```python
from build123d import *

# Parameters (mm, degrees)
F0_R     = 3
F0_R_2   = 7.5
F1_DEPTH = 25
F3_ANGLE = 20


with BuildPart() as f1:
    # F0 (on Top) → F1 (new body)
    with BuildSketch(Plane.XY):
        with BuildLine():
            Line((3, 24.819347), (2, 29.933259))
            Line((2, 29.933259), (-2, 29.933259))
            Line((-2, 29.933259), (-3, 24.819347))
            ThreePointArc((-3, 24.819347), (-4.877258, 24.519632), (-6.726314, 24.078137))
            Line((-6.726314, 24.078137), (-9.607203, 28.420092))
            Line((-9.607203, 28.420092), (-13.302721, 26.889359))
            Line((-13.302721, 26.889359), (-12.269592, 21.782037))
            ThreePointArc((-12.269592, 21.782037), (-13.889256, 20.78674), (-15.428608, 19.671249))
            Line((-15.428608, 19.671249), (-19.751797, 22.580224))
            Line((-19.751797, 22.580224), (-22.580224, 19.751797))
            Line((-22.580224, 19.751797), (-19.671249, 15.428609))
            ThreePointArc((-19.671249, 15.428609), (-20.78674, 13.889256), (-21.782037, 12.269592))
            Line((-21.782037, 12.269592), (-26.889359, 13.302722))
            Line((-26.889359, 13.302722), (-28.420092, 9.607203))
            Line((-28.420092, 9.607203), (-24.078137, 6.726315))
            ThreePointArc((-24.078137, 6.726315), (-24.519632, 4.877258), (-24.819347, 3))
            Line((-24.819347, 3), (-29.933259, 2))
            Line((-29.933259, 2), (-29.933259, -2))
            Line((-29.933259, -2), (-24.819347, -3))
            ThreePointArc((-24.819347, -3), (-24.519632, -4.877258), (-24.078137, -6.726314))
            Line((-24.078137, -6.726314), (-28.420092, -9.607203))
            Line((-28.420092, -9.607203), (-26.889359, -13.302721))
            Line((-26.889359, -13.302721), (-21.782037, -12.269592))
            ThreePointArc((-21.782037, -12.269592), (-20.78674, -13.889256), (-19.671249, -15.428608))
            Line((-19.671249, -15.428608), (-22.580224, -19.751797))
            Line((-22.580224, -19.751797), (-19.751797, -22.580224))
            Line((-19.751797, -22.580224), (-15.428608, -19.671249))
            ThreePointArc((-15.428608, -19.671249), (-13.889256, -20.78674), (-12.269592, -21.782037))
            Line((-12.269592, -21.782037), (-13.302721, -26.889359))
            Line((-13.302721, -26.889359), (-9.607203, -28.420092))
            Line((-9.607203, -28.420092), (-6.726314, -24.078137))
            ThreePointArc((-6.726314, -24.078137), (-4.877258, -24.519632), (-3, -24.819347))
            Line((-3, -24.819347), (-2, -29.933259))
            Line((-2, -29.933259), (2, -29.933259))
            Line((2, -29.933259), (3, -24.819347))
            ThreePointArc((3, -24.819347), (4.877258, -24.519632), (6.726314, -24.078137))
            Line((6.726314, -24.078137), (9.607203, -28.420092))
            Line((9.607203, -28.420092), (13.302721, -26.889359))
            Line((13.302721, -26.889359), (12.269592, -21.782037))
            ThreePointArc((12.269592, -21.782037), (13.889256, -20.78674), (15.428608, -19.671249))
            Line((15.428608, -19.671249), (19.751797, -22.580224))
            Line((19.751797, -22.580224), (22.580224, -19.751797))
            Line((22.580224, -19.751797), (19.671249, -15.428608))
            ThreePointArc((19.671249, -15.428608), (20.78674, -13.889256), (21.782037, -12.269592))
            Line((21.782037, -12.269592), (26.889359, -13.302721))
            Line((26.889359, -13.302721), (28.420092, -9.607203))
            Line((28.420092, -9.607203), (24.078137, -6.726314))
            ThreePointArc((24.078137, -6.726314), (24.519632, -4.877258), (24.819347, -3))
            Line((24.819347, -3), (29.933259, -2))
            Line((29.933259, -2), (29.933259, 2))
            Line((29.933259, 2), (24.819347, 3))
            ThreePointArc((24.819347, 3), (24.519632, 4.877258), (24.078137, 6.726314))
            Line((24.078137, 6.726314), (28.420092, 9.607203))
            Line((28.420092, 9.607203), (26.889359, 13.302721))
            Line((26.889359, 13.302721), (21.782037, 12.269592))
            ThreePointArc((21.782037, 12.269592), (20.78674, 13.889256), (19.671249, 15.428608))
            Line((19.671249, 15.428608), (22.580224, 19.751797))
            Line((22.580224, 19.751797), (19.751797, 22.580224))
            Line((19.751797, 22.580224), (15.428608, 19.671249))
            ThreePointArc((15.428608, 19.671249), (13.889256, 20.78674), (12.269592, 21.782037))
            Line((12.269592, 21.782037), (13.302721, 26.889359))
            Line((13.302721, 26.889359), (9.607203, 28.420092))
            Line((9.607203, 28.420092), (6.726314, 24.078137))
            ThreePointArc((6.726314, 24.078137), (4.877258, 24.519632), (3, 24.819347))
        make_face()
        with Locations((5.212864, -15)):
            Circle(F0_R, mode=Mode.SUBTRACT)
        Circle(F0_R_2, mode=Mode.SUBTRACT)
        with Locations((0, 15)):
            Circle(F0_R, mode=Mode.SUBTRACT)
    extrude(amount=F1_DEPTH)


with BuildPart() as f1_1:
    # F3: moved
    add(f1.part.rotate(Axis((0.748886, 0, 25), (1, 0, 0)), F3_ANGLE))


solid = f1_1.part
```
Model file for the job. Use its own axes, mm. A direction names the side the tool comes from. Give positions to 0.01 mm unless a question says otherwise; leave off trailing zeros. Loops run counter-clockwise (first coordinate to the right, second up) from the corner with the lowest first, then second, coordinate; pieces in that order, holes last. Notation, with made-up numbers: M 89.5,28.5 L 138.5,28.5 A25 ccw 138.5,56.5 Z; hole C 86,67.25 d9. An arc over 180 degrees is marked long. Use one line per item in the form item = value.
Item 1: Slice it at A-A on x = 10.5. List the corners of the cut face in (y, z).
Filled in:
outline = M -26.36,15.41 L -17.81,-8.09 L 34.91,11.1 L 26.36,34.59 Z
Item 2: Which spindle directions (+Z, -Z, +X, -X, +Y, -Y) get a long thin tool onto all of the face, cutting with end or side? Do faces 4 (the flat face through (26.22, 11.99, 15.88)), 5 (the cylindrical face through (-4.85, 27.38, 21.48)), 6 (the flat face through (-27.34, 6.69, 13.95)). Say none if no direction does.
Filled in:
face_4 = +X
face_5 = +Z, +Y
face_6 = -X
Item 3: Two-plate mould, pull along X, no slides. Class faces 1 (the flat face through (-27.644, 15.124, 17.016)), 2 (the flat face through (29.933, 4, 13)), 3 (the flat face through (8.147, -20.302, 4.122)): released by +X, released by -X, zero draft, split by the parting line, or undercut.
Filled in:
face_1 = released by -X
face_2 = released by +X
face_3 = undercut
Item 4: Drill centre lines: L1, parallel to X at y = 22, z = 24.5; L2, parallel to X at y = 9.5, z = 4; L3, parallel to X at y = 31.5, z = 14. Where is each one in solid material? Low to high.
Filled in:
L1 = -21.83 to -16.66, -14.31 to 14.31, 16.66 to 21.83
L2 = -29.93 to -7.29, 7.29 to 29.93
L3 = -13.09 to -7.89, -2.8 to 2.8, 7.89 to 13.09
Item 5: Flat gauge pins, fed straight in: pin 1 Ø6 at (x, y) = (-1, 22.5) entering from -Z; pin 2 Ø8 at (y, z) = (18, 15.5) entering from -X; pin 3 Ø8 at (x, z) = (-12.5, 28) entering from +Y. Where does each tip first touch, or does it go through?
Filled in:
pin_1 = 5.49
pin_2 = -28.4
pin_3 = 30.16
